Geometry check sheet. Reference: drawing and pictorial views, mm from the part's lowest x, y, z. Round coordinates to 2 decimals unless told otherwise and drop trailing zeros. Write each loop counter-clockwise with the first axis right and the second up, starting at its lowest first coordinate (ties: lowest second). Pieces come first, ordered by that corner, then holes. Notation, with made-up numbers: (76, 8.5) -> (119, 8.5) arc R14 ccw to (119, 33.5) -> close; hole circle Ø4 at (-19.5, 32.5). An arc over 180 degrees is marked (long way). Answer as a JSON object with one key per item and string values. Group by question number.
(1) Scan lines: L1, parallel to X at y = 3, z = 4; L2, parallel to Z at x = 296, y = 2.2; L3, parallel to X at y = 19.5, z = 131.5. Record each from-to range of solid material in increasing order. Write a range as from..to.
(2) Sectioned sample at B-B on y = 20. Record the cut outline in (x, z).
(3) Draft check along Z on the marked faces 1, 2 and 3. Enter one of: released by +Z, released by -Z, zero draft, split by the parting line, or undercut.
(4) Sectioned sample at A-A on x = 150. Record the cut outline in (y, z), and give its area (3 significant figures).
(5) Sectioned sample at D-D on x = 87.5. Record the cut outline in (y, z).
(6) Sectioned sample at C-C on z = 100. Record the cut outline in (x, y).
(7) Gauge pin test, flat ends, axial feed: pin 1 Ø21 at (y, z) = (17.5, 112.5) entering from -X; pin 2 Ø8 at (x, y) = (164.5, 17) entering from -Z; pin 3 Ø1 at (x, z) = (159, 68) entering from -Y; pin 4 Ø1.5 at (y, z) = (9, 173) entering from +X. Record the tip position at first contact, or that the pin passes through.
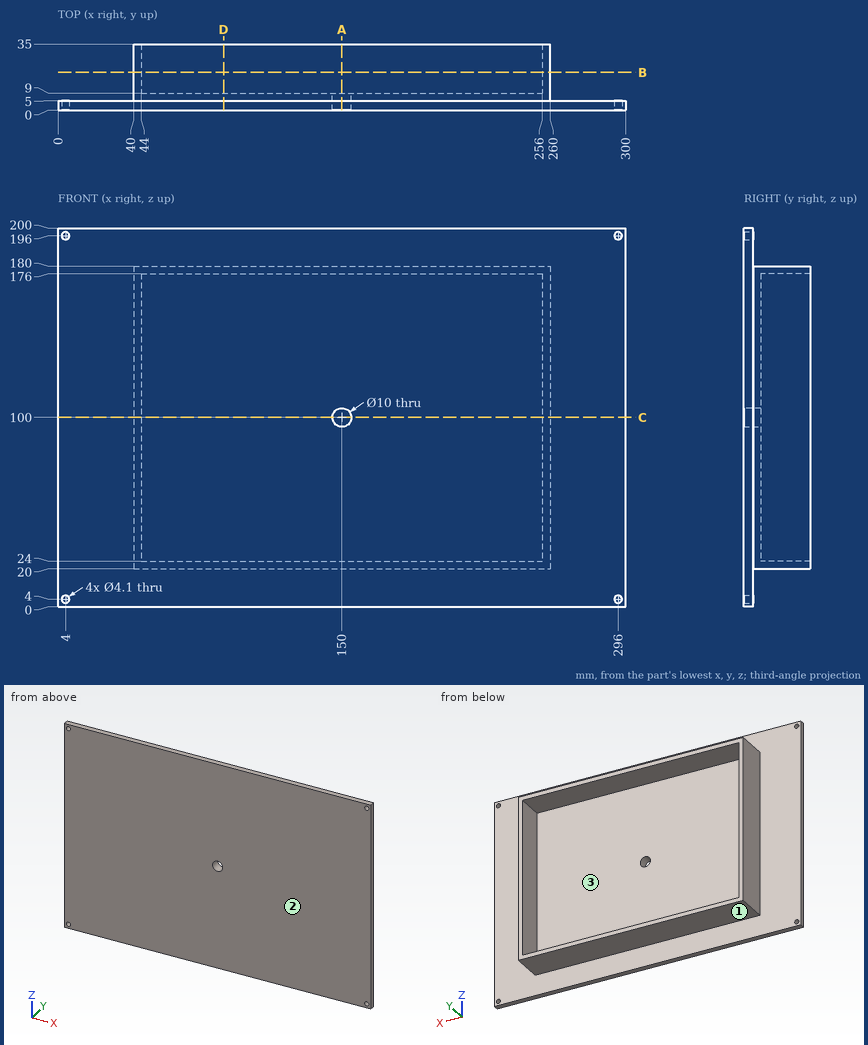
Computed values:
{
 "1": {"L1": "0..1.95, 6.05..293.95, 298.05..300", "L2": "0..1.95, 6.05..193.95, 198.05..200", "L3": "40..44, 256..260"},
 "2": {"outline": "(40, 20) -> (260, 20) -> (260, 180) -> (40, 180) -> close; hole (44, 24) -> (256, 24) -> (256, 176) -> (44, 176) -> close"},
 "3": {"face 1": "released by -Z", "face 2": "zero draft", "face 3": "undercut"},
 "4": {"outline": "(0, 0) -> (5, 0) -> (5, 20) -> (35, 20) -> (35, 24) -> (9, 24) -> (9, 95) -> (0, 95) -> close; (0, 105) -> (9, 105) -> (9, 176) -> (35, 176) -> (35, 180) -> (5, 180) -> (5, 200) -> (0, 200) -> close", "area": "1,760 mm2"},
 "5": {"outline": "(0, 0) -> (5, 0) -> (5, 20) -> (35, 20) -> (35, 24) -> (9, 24) -> (9, 176) -> (35, 176) -> (35, 180) -> (5, 180) -> (5, 200) -> (0, 200) -> close"},
 "6": {"outline": "(0, 0) -> (145, 0) -> (145, 9) -> (44, 9) -> (44, 35) -> (40, 35) -> (40, 5) -> (0, 5) -> close; (155, 0) -> (300, 0) -> (300, 5) -> (260, 5) -> (260, 35) -> (256, 35) -> (256, 9) -> (155, 9) -> close"},
 "7": {"pin 1": "x = 40", "pin 2": "z = 20", "pin 3": "y = 0", "pin 4": "x = 260"}
}
